```python
from build123d import *

# Parameters (mm, degrees)
BOSS_EXTRUDE2_DEPTH = 23
BOSS_EXTRUDE3_DEPTH = 54
CUT_EXTRUDE1_DEPTH  = 27
CUT_EXTRUDE3_DEPTH  = 127.368508735
SKETCH8_W           = 26
SKETCH8_H           = 26
CUT_EXTRUDE4_DEPTH  = 10
SKETCH9_R           = 6
CUT_EXTRUDE5_DEPTH  = 127.368508735
SKETCH10_R          = 4
CUT_EXTRUDE7_DEPTH  = 52
CHAMFER2_SIZE       = 1
FILLET1_R           = 8


with BuildPart() as part:
    # Sketch1 → Boss-Extrude2 (new, symmetric)
    with BuildSketch(Plane.XY):
        Polygon((-104, 0), (104, 0), (99.985564599, 14), (-99.985564599, 14), align=None)
    extrude(amount=BOSS_EXTRUDE2_DEPTH, both=True)

    # Sketch3 → Boss-Extrude3 (add)
    with BuildSketch(Plane(origin=(0, 14, 0), x_dir=(1, 0, 0), z_dir=(0, 1, 0))):
        with BuildLine():
            ThreePointArc((51.058789645, -23), (56, 0), (51.058789645, 23))
            Line((51.058789645, 23), (-51.058789645, 23))
            ThreePointArc((-51.058789645, 23), (-56, 0), (-51.058789645, -23))
            Line((-51.058789645, -23), (51.058789645, -23))
        make_face()
    extrude(amount=BOSS_EXTRUDE3_DEPTH)

    # Sketch5 → Cut-Extrude1 (cut, symmetric)
    with BuildSketch(Plane.XY):
        with BuildLine():
            Line((-28, 75.269278216), (-28, 52))
            Line((-28, 52), (-23.664319132, 52))
            ThreePointArc((-23.664319132, 52), (0, 24), (23.664319132, 52))
            Line((23.664319132, 52), (28, 52))
            Line((28, 52), (28, 75.269278216))
            Line((28, 75.269278216), (-28, 75.269278216))
        make_face()
    extrude(amount=CUT_EXTRUDE1_DEPTH, both=True, mode=Mode.SUBTRACT)

    # Sketch6 → Cut-Extrude3 (cut, through all)
    with BuildSketch(Plane(origin=(0, 68, 0), x_dir=(1, 0, 0), z_dir=(0, 1, 0))):
        with BuildLine():
            Line((-85, 6), (-77, 6))
            ThreePointArc((-77, 6), (-71, 0), (-77, -6))
            Line((-77, -6), (-85, -6))
            ThreePointArc((-85, -6), (-91, 0), (-85, 6))
        make_face()
        with BuildLine():
            Line((77, 6), (85, 6))
            ThreePointArc((85, 6), (91, 0), (85, -6))
            Line((85, -6), (77, -6))
            ThreePointArc((77, -6), (71, 0), (77, 6))
        make_face()
    extrude(amount=-CUT_EXTRUDE3_DEPTH, mode=Mode.SUBTRACT)

    # Sketch8 → Cut-Extrude4 (cut)
    with BuildSketch(Plane.XZ):
        with Locations((39, 0)):
            Rectangle(SKETCH8_W, SKETCH8_H)
        with Locations((-39, 0)):
            Rectangle(SKETCH8_W, SKETCH8_H)
    extrude(amount=-CUT_EXTRUDE4_DEPTH, mode=Mode.SUBTRACT)

    # Sketch9 → Cut-Extrude5 (cut, through all)
    with BuildSketch(Plane.XZ):
        with Locations(Location((-39, 0, 0), (0, 0, 270))):
            Circle(SKETCH9_R)
        with Locations(Location((39, 0, 0), (0, 0, 90))):
            Circle(SKETCH9_R)
    extrude(amount=-CUT_EXTRUDE5_DEPTH, mode=Mode.SUBTRACT)

    # Sketch10 → Cut-Extrude7 (cut)
    with BuildSketch(Plane(origin=(0, 14, 0), x_dir=(1, 0, 0), z_dir=(0, 1, 0))):
        with Locations(Location((0, 0, 0), (0, 0, 90))):
            Circle(SKETCH10_R)
    extrude(amount=CUT_EXTRUDE7_DEPTH, mode=Mode.SUBTRACT)

    # Chamfer2
    chamfer2_edges = [part.edges().sort_by_distance(p)[0] for p in [
        (81, 14, 6),
        (91, 14, 0),
        (81, 14, -6),
        (71, 14, 0),
        (-91, 14, 0),
        (-81, 14, -6),
        (-71, 14, 0),
        (-81, 14, 6),
    ]]
    chamfer(chamfer2_edges, length=CHAMFER2_SIZE)

    # Fillet1
    fillet1_edges = [part.edges().sort_by_distance(p)[0] for p in [
        (56, 14, 0),
        (-56, 14, 0),
    ]]
    fillet(fillet1_edges, radius=FILLET1_R)


solid = part.part
```
For this review, take the finished solid that the model builds, in its own axes (mm). A direction names the side the tool comes from. Give positions to 0.01 mm unless a question says otherwise; leave off trailing zeros. Loops run counter-clockwise (first coordinate to the right, second up) from the corner with the lowest first, then second, coordinate; pieces in that order, holes last. Notation, with made-up numbers: M 10,33.25 L 23,33.25 A22 ccw 23,71.25 Z; hole C 73,32 d2. An arc over 180 degrees is marked long. One line per item, written item: value. Start each with the question number.
Q1. For L1, parallel to X at y = 55, z = 0; L2, parallel to Z at x = 39, y = 47; L3, parallel to X at y = 21, z = 0, list the stretches that pass through material, from the lowest coordinate up.
Q2. Add section A-A (y = 48). Give the boundary of the cut face in (x, z), and give its area (3 significant figures).
Q3. Add section D-D (y = 33.5). Give the boundary of the cut face in (x, z).
Q4. Clearance check with flat-ended pins moving along their axes: pin 1 Ø17.5 at (y, z) = (58, -6.5) entering from -X; pin 2 Ø2 at (x, z) = (25.5, -2.5) entering from +Y; pin 3 Ø1 at (x, z) = (70, 14) entering from +Y. State where each tip first meets the part, or that it passes through.
Q5. Add section B-B (x = -39). Give the boundary of the cut face in (y, z), and give its area (3 significant figures).
Q6. Add section C-C (z = 0). Count the separate pieces of the cut face and the enclosed holes in it, and give its area (3 significant figures).
Q7. Machinability: for faces 1 (the face through (33, 10, 3)), 2 (the face through (56, 45, 0)), 3 (the face through (91.2, 13.2, -0.1)), 4 (the face through (91, 7, 0)), which of the approach directions +Z, -Z, +X, -X, +Y, -Y give a long, thin tool a straight path to every point of the face, cutting with its end or side? Answer none if there is none.
Q8. Draft analysis for pull direction Z (two halves, no side actions). For faces 5 (the face through (26, 5, 0)), 6 (the face through (-45.3, 68, -0.3)), 7 (the face through (-1, 19, 23)), state which applies: released by +Z, released by -Z, zero draft, split by the parting line, or undercut.
Reply:
1. L1: -56 to -45, -33 to -28, 28 to 33, 45 to 56
1. L2: -23 to -6, 6 to 23
1. L3: -56.06 to -45, -33 to -4, 4 to 33, 45 to 56.06
2. outline: M -51.06,-23 L -24,-23 L -24,23 L -51.06,23 A56 ccw Z; M 24,-23 L 51.06,-23 A56 ccw 51.06,23 L 24,23 Z; hole C -39,0 d12; hole C 39,0 d12
2. area: 2,570 mm²
3. outline: M -51.06,-23 L -19.12,-23 L -19.12,23 L -51.06,23 A56 ccw Z; M 19.12,-23 L 51.06,-23 A56 ccw 51.06,23 L 19.12,23 Z; hole C -39,0 d12; hole C 39,0 d12
4. pin 1: x = -56
4. pin 2: y = 52
4. pin 3: y = 14
5. outline: M 0,-23 L 68,-23 L 68,-6 L 10,-6 L 10,-13 L 0,-13 Z; M 0,13 L 10,13 L 10,6 L 68,6 L 68,23 L 0,23 Z
5. area: 2,170 mm²
6. separate pieces: 5
6. enclosed holes: 0
6. area: 4,380 mm²
7. face 1: -Y
7. face 2: +X, +Y
7. face 3: +Y
7. face 4: +Y, -Y
8. face 5: undercut
8. face 6: zero draft
8. face 7: released by +Z
